Autodesk Inventor part; units mm, degrees
ref_plane "YZ Plane" through (0, 0, 0) normal (1, 0, 0) x (0, 1, 0)
ref_plane "XZ Plane" through (0, 0, 0) normal (0, 1, 0) x (-1, 0, 0)
ref_plane "XY Plane" through (0, 0, 0) normal (0, 0, 1) x (1, 0, 0)
sketch "Sketch1" plane through (0, 0, 0) normal (0, 1, 0) x (-1, 0, 0)
  line L0 (12, 0) -> (-66.5, 0)
  line L1 (-66.5, 0) -> (-66.5, -61.3)
  line L2 (-66.5, -61.3) -> (12, -61.3)
  line L3 (12, -61.3) -> (12, 0)
  point P0 (0, 0)
  dimension "d0" = 12
  dimension "d1" = 66.5
  dimension "d2" = 61.3
extrude "Extrusion1" add sketch "Sketch1" against normal blind 12
sketch "Sketch2" plane through (0, 0, 0) normal (0, 1, 0) x (1, 0, 0)
  line L0 (61.5, 56.5) -> (10, 56.5)
  line L1 (10, 56.5) -> (10, 5)
  line L2 (10, 5) -> (61.5, 5)
  line L3 (61.5, 5) -> (61.5, 56.5)
  line L4 (-12, 0) -> (66.5, 0)
  point P0 (0, 0)
  dimension "d5" = 10
  dimension "d6" = 51.5
  dimension "d7" = 5
  dimension "d8" = 51.5
extrude "Extrusion2" cut sketch "Sketch2" against normal blind 6.2
sketch "Sketch3" plane through (0, 0, 0) normal (0, 1, 0) x (1, 0, 0)
  line L0 (61.5, 5) -> (10, 5)
  circle A0 centre (10, 5) radius 1.5
  circle A1 centre (61.5, 5) radius 1.5
  line L1 (10, 56.5) -> (61.5, 56.5)
  circle A2 centre (61.5, 56.5) radius 1.5
  circle A3 centre (10, 56.5) radius 1.5
  point P0 (0, 0)
  dimension "d11" = 3
extrude "Extrusion3" cut sketch "Sketch3" against normal through all
chamfer "Chamfer1" distance 0.8 angle 45 8 edges at (10, -3.1, -6.5) (10, -3.1, -55) (11.5, -3.1, -56.5) (60, -3.1, -56.5) (61.5, -3.1, -55) (61.5, -3.1, -6.5) (60, -3.1, -5) (11.5, -3.1, -5)
sketch "Sketch4" plane through (0, -6.2, 0) normal (0, 1, 0) x (1, 0, 0)
  arc A0 (9.229, 55.2133) -> (11.2867, 57.271) centre (10, 56.5) ccw construction
  line L0 (10, 56.5) -> (61.5, 56.5) construction
  line L1 (61.5, 56.5) -> (61.5, 5) construction
  line L2 (61.5, 5) -> (10, 5) construction
  line L3 (10, 5) -> (10, 56.5) construction
  arc A1 (60.2133, 4.229) -> (62.271, 6.2867) centre (61.5, 5) ccw construction
  line L4 (58.5, 8) -> (58.5, 53.5) construction
  line L5 (58.5, 53.5) -> (13, 53.5) construction
  line L6 (13, 53.5) -> (13, 8) construction
  line L7 (13, 8) -> (58.5, 8) construction
  line L8 (13, 8) -> (58.5, 8)
  line L9 (58.5, 8) -> (58.5, 53.5)
  line L10 (58.5, 53.5) -> (13, 53.5)
  line L11 (13, 53.5) -> (13, 8)
  point P0 (0, 0)
  dimension "d19" = 3
extrude "Extrusion4" cut sketch "Sketch4" against normal blind 6.2
fillet "Fillet1" radius 3 4 edges at (13, -9.1, -53.5) (58.5, -9.1, -8) (13, -9.1, -8) (58.5, -9.1, -53.5)
sketch "Sketch5" plane through (66.5, 0, -61.3) normal (0, 0, -1) x (-1, 0, 0)
  line L0 (0, 0) -> (78.5, 0)
  point P0 (66.5, 0)
  point P1 (31.1, -3.5)
  point P2 (56.5, -6.2)
  dimension "d24" = 25.4
  dimension "d25" = 3.5
hole "Hole1" at (35.4, -3.5, -61.3) direction (0, 0, 1) diameter 2.459 depth 8.8 tip angle 118
chamfer "Chamfer2" [suppressed]
sketch "Sketch6" plane through (-12, 0, -61.3) normal (-1, 0, 0) x (0, 0, 1)
  line L0 (56.3, 0) -> (56.3, -6.2)
  line L1 (56.3, -6.2) -> (56.3, 0)
  line L2 (4.8, -2.2705) -> (4.8, -4.7295)
  line L3 (4.8, 0) -> (4.8, -6.2)
  line L4 (4.8, -6.2) -> (4.8, 0)
  line L5 (30.9, -24.2917) -> (30.9, 19.2353) construction
  line L6 (49.4, 0) -> (12.4, 0) construction
  line L7 (12.4, 0) -> (12.4, -12) construction
  line L8 (12.4, -12) -> (49.4, -12) construction
  line L9 (49.4, -12) -> (49.4, 0) construction
  line L10 (49.4, 0) -> (12.4, -12) construction
  line L11 (12.4, 0) -> (49.4, -12) construction
  line L12 (0, 0) -> (61.3, 0)
  line L13 (61.3, -12) -> (0, -12)
  line L14 (7.1, -6.2) -> (54, -6.2)
  point P0 (30.9, -6)
  point P1 (19.7, -6.2)
  point P2 (42.1, -6.2)
  dimension "d36" = 25.4
  dimension "d37" = 37
  dimension "d38" = 22.4
hole "Hole2" at (-12, -6.2, -41.6) at (-12, -6.2, -19.2) at (-12, -6, -30.4) direction (1, 0, 0) diameter 3.242 depth 11.8 tip angle 118
sketch "Sketch7" plane through (-12, 0, 0) normal (0, 0, 1) x (1, 0, 0)
  line L0 (0, 0) -> (78.5, 0)
  line L1 (16.5, -4.5) -> (7.5, -4.5) construction
  point P0 (12, 0)
  dimension "d52" = 9
  dimension "d53" = 4.5
  dimension "d54" = 4.5
hole "Hole3" at (-4.5, -4.5, 0) at (4.5, -4.5, 0) direction (0, 0, -1) diameter 3.242 depth 11.8 tip angle 118
properties part number "MirrorHolder" material "Aluminum 6061"
Input: part model. Units: mm. Frame: model coordinates. A direction names the side the tool comes from. Coordinates: 2 decimals unless noted, no trailing zeros. Loops run counter-clockwise (first coordinate to the right, second up) from the corner with the lowest first, then second, coordinate; pieces in that order, holes last. Notation, with made-up numbers: M -38,-5 L 13,-5 A20 cw 13,29 Z; hole C -24.5,23 d9. An arc over 180 degrees is marked long. Answer in a Markdown table with one row per item.
1. Section B-B, the plane z = -25. Output: boundary loops of the cut face in (x, y).
Response:
| item | result |
|---|---|
| outline | M -12,-12 L 13,-12 L 13,-6.2 L 10,-6.2 L 10,0 L -12,0 Z; M 58.5,-12 L 66.5,-12 L 66.5,0 L 61.5,0 L 61.5,-6.2 L 58.5,-6.2 Z |
2. Section A-A, the plane x = 27. Output: boundary loops of the cut face in (y, z), then the cut area to 3 significant figures.
Response:
| item | result |
|---|---|
| outline | M -12,-61.3 L 0,-61.3 L 0,-56.5 L -6.2,-56.5 L -6.2,-53.5 L -12,-53.5 Z; M -12,-8 L -6.2,-8 L -6.2,-5 L 0,-5 L 0,0 L -12,0 Z |
| area | 152 mm2 |
3. First-contact query: pin 1 (3.5 mm diameter, centred on x = -4.5, y = -4.5, fed in from +Z); pin 2 (1.9 mm diameter, centred on y = -6, z = -30.4, fed in from -X); pin 3 (1.9 mm diameter, centred on x = 4.5, y = -4.5, fed in from +Z). Flat tips, straight axial feed; report the tip coordinate or a pass-through.
Response:
| item | result |
|---|---|
| pin 1 | stops at z = 0 |
| pin 2 | stops at x = 0.2 |
| pin 3 | stops at z = -12.2 |
4. Reachability of faces 1 (the flat face through (58.5, -9, -30)), 2 (the flat face through (61.5, -3, -30)), 3 (the cylindrical face through (5.938, -5.248, -5.983)) from +Z, -Z, +X, -X, +Y, -Y: full face, straight path, thin tool, end or side. Return the list, or none.
Response:
| item | result |
|---|---|
| face 1 | +Y, -Y |
| face 2 | +Y |
| face 3 | +Z |
5. Section C-C, the plane y = -10.25. Output: boundary loops of the cut face in (x, z), then the cut area to 3 significant figures.
Response:
| item | result |
|---|---|
| outline | M -12,-61.3 L 66.5,-61.3 L 66.5,0 L -12,0 Z; hole C 10,-56.5 d3; hole C 10,-5 d3; hole M 13,-50.5 A3 ccw 16,-53.5 L 55.5,-53.5 A3 ccw 58.5,-50.5 L 58.5,-11 A3 ccw 55.5,-8 L 16,-8 A3 ccw 13,-11 Z; hole C 61.5,-56.5 d3; hole C 61.5,-5 d3 |
| area | 2,720 mm2 |
6. Material intervals for line 1 (Z direction, x = -9.5, y = -6.2); line 2 (Z direction, x = 10, y = -7.75); line 3 (X direction, y = -4.5, z = -7.5), sorted ascending.
Response:
| item | result |
|---|---|
| line 1 | z = -61.3 to -43.22, -39.98 to -32.01, -28.79 to -20.82, -17.58 to 0 |
| line 2 | z = -61.3 to -58, -55 to -6.5, -3.5 to 0 |
| line 3 | x = -12 to -6.12, -2.88 to 2.88, 6.12 to 10, 61.5 to 66.5 |
7. Section D-D, the plane x = 35.4. Output: boundary loops of the cut face in (y, z).
Response:
| item | result |
|---|---|
| outline | M -12,-61.3 L -4.73,-61.3 L -4.73,-56.5 L -6.2,-56.5 L -6.2,-53.5 L -12,-53.5 Z; M -12,-8 L -6.2,-8 L -6.2,-5 L 0,-5 L 0,0 L -12,0 Z; M -2.27,-61.3 L 0,-61.3 L 0,-56.5 L -2.27,-56.5 Z |
8. Draft query along X for faces 4 (the flat face through (-12, -3, -31)), 5 (the flat face through (12, -6.2, -31)), 6 (the flat face through (66.5, -6, -30)), 7 (the flat face through (10, -3, -31)). Return one class per face: pulls with the +X half, pulls with the -X half, needs draft (parallel to the pull), parting line crosses it, or undercut.
Response:
| item | result |
|---|---|
| face 4 | pulls with the -X half |
| face 5 | undercut |
| face 6 | pulls with the +X half |
| face 7 | undercut |
